Source: three-view drawing plus pictorial views. Frame: mm from the lowest corner of the part. A direction names the side the tool comes from. Coordinates: 2 decimals unless noted, no trailing zeros. Loops run counter-clockwise (first coordinate to the right, second up) from the corner with the lowest first, then second, coordinate; pieces in that order, holes last. Notation, with made-up numbers: M 22.5,89.5 L 33.5,89.5 A4 cw 33.5,93.5 Z; hole C 67,28 d2. An arc over 180 degrees is marked long. Write each question's results on one line, items separated by ' | '. Start each with the question number.
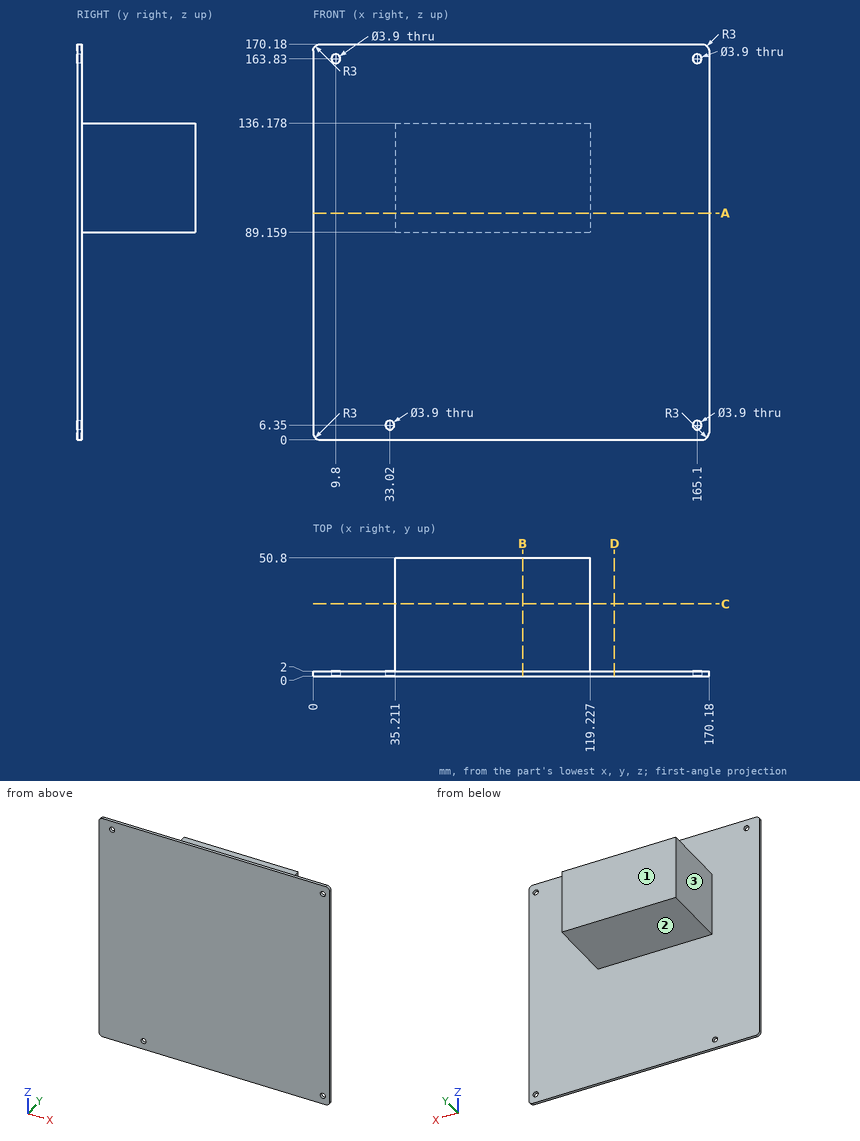
Item 1: Set-up query: the marked faces 1, 2 and 3. Return all of +Z, -Z, +X, -X, +Y, -Y with unobstructed straight access to the full face (end or side cutting, diameter ignored); none if empty.
Item 2: Section D-D, the plane x = 129.5. Return loops of the section in (y, z).
Item 3: Section C-C, the plane y = 31. Return loops of the section in (x, z).
Item 4: Section A-A, the plane z = 97.5. Return loops of the section in (x, y), plus the area to 3 significant figures.
Item 5: Section B-B, the plane x = 90. Return loops of the section in (y, z).
Item 6: Ray query, L1, parallel to X at y = 1.55, z = 163.83; L2, parallel to Z at x = 165.1, y = 1.2; L3, parallel to Z at x = 9.8, y = 0.8. Return the intervals inside material, ascending. Write a range as [from, to].
Item 7: Contact query for flat-ended pins moving along their axis: P1, Ø4, axis at y = 30, z = 139.5, coming from the +X side; P2, Ø12, axis at x = 119.5, y = 44.5, coming from the -Z side; P3, Ø1, axis at y = 34, z = 130.5, coming from the +X side; P4, Ø10, axis at x = 139, z = 150.5, coming from the +Y side. Output: stop coordinate, or through.
Solutions:
1) face 1: +Z, -Z, +X, -X, +Y | face 2: -Z, +X, -X, +Y | face 3: +Z, -Z, -X, +Y
2) outline: M 0,0 L 2,0 L 2,170.18 L 0,170.18 Z
3) outline: M 35.21,89.16 L 119.23,89.16 L 119.23,136.18 L 35.21,136.18 Z
4) outline: M 0,0 L 170.18,0 L 170.18,2 L 119.23,2 L 119.23,50.8 L 35.21,50.8 L 35.21,2 L 0,2 Z | area: 4,440 mm²
5) outline: M 0,0 L 2,0 L 2,89.16 L 50.8,89.16 L 50.8,136.18 L 2,136.18 L 2,170.18 L 0,170.18 Z
6) L1: x = [0, 7.85], [11.75, 163.15], [167.05, 170.18] | L2: z = [0, 4.4], [8.3, 161.88], [165.78, 170.18] | L3: z = [0, 161.88], [165.78, 170.18]
7) P1: passes through | P2: stops at z = 89.16 | P3: stops at x = 119.23 | P4: stops at y = 2
